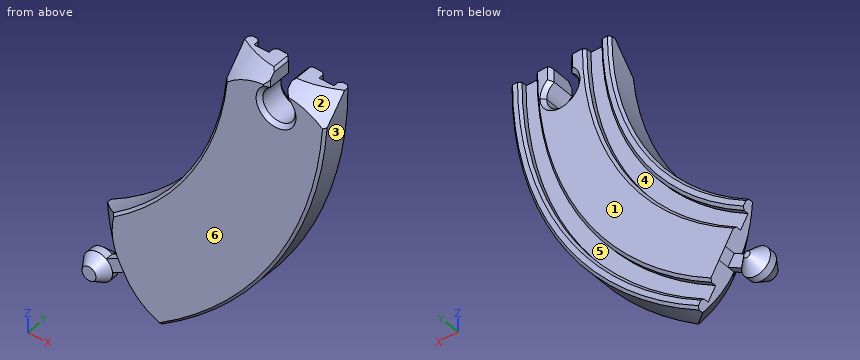
from build123d import *
from build123d.topology import SkipClean

# Parameters (mm, degrees)
REVOLVE1_ANGLE       = 60
CUT_EXTRUDE1_DEPTH   = 151.383351548
BOSS_EXTRUDE1_DEPTH  = 12
BOSS_EXTRUDE2_DEPTH  = 7.5
CUT_EXTRUDE2_DEPTH   = 4.5
CHAMFER2_SIZE        = 4.5
CHAMFER5_SIZE        = 4.5
CHAMFER5_SIZE_2      = 3
CHAMFER3_SIZE        = 1.5
CUT_REVOLVE1_ANGLE   = 90
CHAMFER4_SIZE        = 4.5
MIRROR4_COPY_1_ANGLE = 90
CHAMFER1_SIZE        = 1


# Some blends are built 0.0001 mm under size
with BuildPart() as part:
    # Sketch2 → Revolve1 (revolve)
    with BuildSketch(Plane.XY):
        Polygon((-16, 12), (-20, 12), (-20, 0), (20, 0), (20, 12), (16, 12), (16, 9), (10, 9), (10, 12), (-10, 12), (-10, 9), (-16, 9), align=None)
    revolve(axis=Axis((-129.903810568, 0, 0), (0, 1, 0)), revolution_arc=REVOLVE1_ANGLE)

    # Sketch3 → Cut-Extrude1 (cut, through all)
    with BuildSketch(Plane(origin=(0, 12, 0), x_dir=(1, 0, 0), z_dir=(0, 1, 0))):
        with BuildLine():
            ThreePointArc((6.5, 11.5), (-3.122498999, 17.200877125), (-3.5, 6.022774425))
            Line((-3.5, 6.022774425), (-3.5, 11.5))
            Line((-3.5, 11.5), (3.5, 11.5))
            Line((3.5, 11.5), (3.5, 6.022774425))
            ThreePointArc((3.5, 6.022774425), (5.700877125, 8.377501001), (6.5, 11.5))
        make_face()
        with BuildLine():
            Line((-3.5, 11.5), (-3.5, 6.022774425))
            ThreePointArc((-3.5, 6.022774425), (0, 5), (3.5, 6.022774425))
            Line((3.5, 6.022774425), (3.5, 11.5))
            Line((3.5, 11.5), (-3.5, 11.5))
        make_face()
        with BuildLine():
            Line((-3.5, 6.022774425), (-3.5, 0))
            Line((-3.5, 0), (3.5, 0))
            Line((3.5, 0), (3.5, 6.022774425))
            ThreePointArc((3.5, 6.022774425), (0, 5), (-3.5, 6.022774425))
        make_face()
    extrude(amount=-CUT_EXTRUDE1_DEPTH, mode=Mode.SUBTRACT)



with BuildPart() as body_2:
    # Sketch4 → Boss-Extrude1 (new body)
    with BuildSketch(Plane(origin=(0, 12, 0), x_dir=(1, 0, 0), z_dir=(0, 1, 0))):
        with BuildLine():
            ThreePointArc((-71.628813948, 113.468163669), (-69.888250085, 115.35), (-69.128813948, 117.798290688))
            Line((-69.128813948, 117.798290688), (-73.661197427, 120.415063509))
            Line((-73.661197427, 120.415063509), (-76.161197427, 116.084936491))
            Line((-76.161197427, 116.084936491), (-71.628813948, 113.468163669))
        make_face()
        with BuildLine():
            Line((-73.661197427, 120.415063509), (-69.128813948, 117.798290688))
            ThreePointArc((-69.128813948, 117.798290688), (-69.115603231, 118.023973649), (-69.111197427, 118.25))
            ThreePointArc((-69.111197427, 118.25), (-80.043342407, 120.952052537), (-71.628813948, 113.468163669))
            Line((-71.628813948, 113.468163669), (-76.161197427, 116.084936491))
            Line((-76.161197427, 116.084936491), (-73.661197427, 120.415063509))
        make_face()
    extrude(amount=-BOSS_EXTRUDE1_DEPTH)


with BuildPart() as part_1:
    add(part.part)

    add(body_2.part)  # Boss-Extrude2 merges body 2
    # Sketch4<3> → Boss-Extrude2 (add)
    with BuildSketch(Plane(origin=(0, 12, 0), x_dir=(1, 0, 0), z_dir=(0, 1, 0))):
        with BuildLine():
            Line((-66.201905284, 110.334936491), (-63.701905284, 114.665063509))
            Line((-63.701905284, 114.665063509), (-69.128813948, 117.798290688))
            ThreePointArc((-69.128813948, 117.798290688), (-69.888250085, 115.35), (-71.628813948, 113.468163669))
            Line((-71.628813948, 113.468163669), (-66.201905284, 110.334936491))
        make_face()
    extrude(amount=-BOSS_EXTRUDE2_DEPTH)

    # Sketch4<5> → Cut-Extrude2 (cut)
    with SkipClean():  # the faces are left unmerged after this step: merging them gives an invalid solid
        with BuildSketch(Plane(origin=(0, 12, 0), x_dir=(1, 0, 0), z_dir=(0, 1, 0))):
            with BuildLine():
                Line((-66.201905284, 110.334936491), (-63.701905284, 114.665063509))
                Line((-63.701905284, 114.665063509), (-69.128813948, 117.798290688))
                ThreePointArc((-69.128813948, 117.798290688), (-69.888250085, 115.35), (-71.628813948, 113.468163669))
                Line((-71.628813948, 113.468163669), (-66.201905284, 110.334936491))
            make_face()
        extrude(amount=-CUT_EXTRUDE2_DEPTH, mode=Mode.SUBTRACT)

    # Chamfer2
    chamfer2_edges = [part_1.edges().sort_by_distance(p)[0] for p in [
        (-79.934144769, 12, -121.15),
    ]]
    chamfer(chamfer2_edges, length=CHAMFER2_SIZE - 0.0001)  # a hair under: the kernel refuses the full size

    # Chamfer5
    # the kernel refuses this chamfer: 4.5, 3 mm, written as the material it takes off along each edge
    with BuildSketch(Plane(origin=(-74.911197427, 0, -118.25), x_dir=(0.5659281860209275, 1.3089718800099638e-15, 0.8244545398425934), z_dir=(-0.8244545398425934, -1.906934193520804e-15, 0.5659281860209275))) as chamfer5_piece_1:
        Polygon((5.8, CHAMFER5_SIZE), (5.8 - CHAMFER5_SIZE_2, 0), (5.8, 0), align=None)
    revolve(axis=Axis((-74.911197427, 0, -118.25), (0, 1, 0)), mode=Mode.SUBTRACT)

    # Chamfer3
    chamfer3_edges = [part_1.edges().sort_by_distance(p)[0] for p in [
        (0, 0, -18),
        (3.5, 0, -3.011387212),
        (-3.5, 12, -3.011387212),
        (-3.5, 0, -3.011387212),
        (0, 12, -18),
        (3.5, 12, -3.011387212),
    ]]
    chamfer(chamfer3_edges, length=CHAMFER3_SIZE)

    # Sketch17 → Cut-Revolve1 (revolve, cut)
    with BuildSketch(Plane(origin=(31.225952642, 0, -54.084936491), x_dir=(0.8660254037844438, 0, 0.49999999999999123), z_dir=(-0.49999999999999123, -1.1564823173178522e-15, 0.8660254037844438))):
        Polygon((-118.766454357, 10.766454357), (-118.766454357, 0), (-108, 0), align=None)
    cut_revolve1 = revolve(axis=Axis((-40.654155872, -1.265151723, -95.584936491), (0, 1, 0)), revolution_arc=CUT_REVOLVE1_ANGLE, mode=Mode.SUBTRACT)

    # Mirror1: Cut-Revolve1 across plane
    add(cut_revolve1.mirror(Plane(origin=(32.475952642, 0, -56.25), x_dir=(0.8660254037844437, 2.0030861316495613e-15, 0.4999999999999914), z_dir=(-0.49999999999999156, -1.1564823173178542e-15, 0.8660254037844436))), mode=Mode.SUBTRACT)

    # Chamfer4
    chamfer4_edges = [part_1.edges().sort_by_distance(p)[0] for p in [
        (-64.951905284, 0, -112.5),
    ]]
    chamfer(chamfer4_edges, length=CHAMFER4_SIZE - 0.0001)  # a hair under: the kernel refuses the full size

    # Mirror4: Cut-Revolve1 across plane
    add(cut_revolve1.mirror(Plane(origin=(-32.475952642, 0, -56.25), x_dir=(-0.8660254037844385, -2.0030861316495455e-15, 0.5000000000000006), z_dir=(-0.5000000000000009, -1.1564823173178735e-15, -0.8660254037844383))), mode=Mode.SUBTRACT)

    # Mirror4 copy 1 sketch → Mirror4 copy 1 (revolve, cut)
    with BuildSketch(Plane(origin=(2.5, 0, -112.5), x_dir=(0, 0, -1), z_dir=(1, 0, 0))):
        Polygon((-118.766454357, 10.766454357), (-118.766454357, 0), (-108, 0), align=None)
    revolve(axis=Axis((2.5, -1.265151723, -29.5), (0, 1, 0)), revolution_arc=MIRROR4_COPY_1_ANGLE, mode=Mode.SUBTRACT)

    # Chamfer1
    chamfer1_edges = [part_1.edges().sort_by_distance(p)[0] for p in [
        (-34.724318643, 0, -54.951905284),
        (-0.083302492, 0, -74.951905284),
        (-3.5, 7.508472143, 0),
        (3.5, 7.508472143, 0),
        (-31.260217028, 12, -56.951905284),
        (-26.064064606, 12, -59.951905284),
        (-8.74355653, 12, -69.951905284),
        (-3.547404107, 12, -72.951905284),
        (-0.083302492, 12, -74.951905284),
        (-34.724318643, 12, -54.951905284),
    ]]
    chamfer(chamfer1_edges, length=CHAMFER1_SIZE)


solid = part_1.part
CAD build for the part. Positions are in the model's coordinates, mm. Face numbers are marked on the shaded views. A direction names the side the tool comes from. Give positions to 0.01 mm unless a question says otherwise; leave off trailing zeros. Return JSON: item names as keys, results as strings.
Item 1: Drill centre lines: probe 1 along X at (y, z) = (11.5, -23); probe 2 along X at (y, z) = (6.75, -11.5); probe 3 along X at (y, z) = (10.75, -69.5). Where is each one in solid material? Low to high.
Answer below:
{"probe 1": "x = -21.92 to -18.86, -11.72 to 7.59, 14.68 to 17.72", "probe 2": "x = -20.6 to -6.5, 6.5 to 19.56", "probe 3": "x = -44.77 to -39.66, -32.2 to -8.48, -1.62 to 2.92"}
Item 2: Tool access for the marked faces 5 and 6: list every direction of +Z, -Z, +X, -X, +Y, -Y with a clear straight run to the whole face (end or side of a thin tool).
Answer below:
{"face 5": "+Y", "face 6": "+Z, -Z, +X, -X, -Y"}
Item 3: Two-plate mould, pull along Z, no slides. Class the marked faces 1, 2, 3 and 4: +Z half, -Z half, draft (parallel to the pull), parting line (faces both ways), or undercut.
Answer below:
{"face 1": "draft", "face 2": "+Z half", "face 3": "-Z half", "face 4": "undercut"}
Item 4: Drop flat-ended pins along their axis: pin 1 (6 mm diameter, centred on x = -47, y = 3, fed in from -Z); pin 2 (4 mm diameter, centred on y = 5.5, z = -105.5, fed in from +X); pin 3 (6 mm diameter, centred on y = 2.5, z = -48.5, fed in from +X). Give the stop position or say it passes through.
Answer below:
{"pin 1": "stops at z = -126.68", "pin 2": "stops at x = -21.47", "pin 3": "stops at x = 12.93"}
